Can you work these out from the model? Positions are in its coordinate system, mm. A direction names the side the tool comes from. Coordinates: 2 decimals unless noted, no trailing zeros. Loops run counter-clockwise (first coordinate to the right, second up) from the corner with the lowest first, then second, coordinate; pieces in that order, holes last.
```python
from build123d import *

# Parameters (mm, degrees)
BOSS_EXTRUDE1_DEPTH = 60
SKETCH2_R           = 1.65
SKETCH2_R_2         = 11.5
CUT_EXTRUDE1_DEPTH  = 60
SKETCH3_R           = 1.65
SKETCH3_R_2         = 11.5
CUT_EXTRUDE2_DEPTH  = 60
CUT_EXTRUDE3_START  = -21
SKETCH4_R           = 4
CUT_EXTRUDE3_DEPTH  = 21
SKETCH5_R           = 2.5
CUT_EXTRUDE4_DEPTH  = 6
CUT_EXTRUDE5_DEPTH  = 10
SKETCH9_R           = 5.25
CUT_EXTRUDE7_DEPTH  = 3
CHAMFER1_SIZE       = 1
SKETCH10_W          = 5
SKETCH10_H          = 82
BOSS_EXTRUDE2_DEPTH = 6
FILLET1_R           = 5
SKETCH11_R          = 1.65
CUT_EXTRUDE8_DEPTH  = 10
CUT_EXTRUDE9_DEPTH  = 5
SKETCH13_W          = 82
SKETCH13_H          = 5
BOSS_EXTRUDE3_DEPTH = 6
FILLET2_R           = 5
SKETCH14_R          = 1.5
CUT_EXTRUDE10_DEPTH = 5
CUT_EXTRUDE11_DEPTH = 5


with BuildPart() as part:
    # Sketch1 → Boss-Extrude1 (new body)
    with BuildSketch(Plane(origin=(0, 0, 0), x_dir=(1, 0, 0), z_dir=(0, 1, 0))):
        Polygon((0, 0), (0, -42), (-5, -42), (-5, 40), (0, 40), (0, 5), (82, 5), (82, 0), align=None)
    extrude(amount=BOSS_EXTRUDE1_DEPTH)

    # Sketch2 → Cut-Extrude1 (cut)
    with BuildSketch(Plane.XY):
        with Locations((45.5, 36.5)):
            Circle(SKETCH2_R)
        with Locations((76.5, 36.5)):
            Circle(SKETCH2_R)
        with Locations((76.5, 5.5)):
            Circle(SKETCH2_R)
        with Locations((45.5, 5.5)):
            Circle(SKETCH2_R)
        with Locations((61, 21)):
            Circle(SKETCH2_R_2)
    extrude(amount=-CUT_EXTRUDE1_DEPTH, mode=Mode.SUBTRACT)

    # Sketch3 → Cut-Extrude2 (cut)
    with BuildSketch(Plane(origin=(0, 0, 0), x_dir=(0, 0, -1), z_dir=(1, 0, 0))):
        with Locations((-36.5, 53.5)):
            Circle(SKETCH3_R)
        with Locations((-5.5, 53.5)):
            Circle(SKETCH3_R)
        with Locations((-5.5, 22.5)):
            Circle(SKETCH3_R)
        with Locations((-36.5, 22.5)):
            Circle(SKETCH3_R)
        with Locations((-21, 38)):
            Circle(SKETCH3_R_2)
    extrude(amount=-CUT_EXTRUDE2_DEPTH, mode=Mode.SUBTRACT)

    # Sketch4 → Cut-Extrude3 (cut)
    with BuildSketch(Plane(origin=(0, 0, -5), x_dir=(-1, 0, 0), z_dir=(0, 0, -1)).offset(CUT_EXTRUDE3_START)):
        with Locations((-61, 53)):
            Circle(SKETCH4_R)
        with BuildLine():
            Line((-47.15, 36.5), (-47.15, 41.5))
            ThreePointArc((-47.15, 41.5), (-45.5, 43.15), (-43.85, 41.5))
            Line((-43.85, 41.5), (-43.85, 36.5))
            ThreePointArc((-43.85, 36.5), (-45.5, 34.85), (-47.15, 36.5))
        make_face()
        with BuildLine():
            Line((-78.15, 36.5), (-78.15, 41.5))
            ThreePointArc((-78.15, 41.5), (-76.5, 43.15), (-74.85, 41.5))
            Line((-74.85, 41.5), (-74.85, 36.5))
            ThreePointArc((-74.85, 36.5), (-76.5, 34.85), (-78.15, 36.5))
        make_face()
        with BuildLine():
            Line((-78.15, 5.5), (-78.15, 10.5))
            ThreePointArc((-78.15, 10.5), (-76.5, 12.15), (-74.85, 10.5))
            Line((-74.85, 10.5), (-74.85, 5.5))
            ThreePointArc((-74.85, 5.5), (-76.5, 3.85), (-78.15, 5.5))
        make_face()
        with BuildLine():
            Line((-47.15, 5.5), (-47.15, 10.5))
            ThreePointArc((-47.15, 10.5), (-45.5, 12.15), (-43.85, 10.5))
            Line((-43.85, 10.5), (-43.85, 5.5))
            ThreePointArc((-43.85, 5.5), (-45.5, 3.85), (-47.15, 5.5))
        make_face()
        with BuildLine():
            Line((-72.5, 21), (-72.5, 26))
            ThreePointArc((-72.5, 26), (-61, 37.5), (-49.5, 26))
            Line((-49.5, 26), (-49.5, 21))
            ThreePointArc((-49.5, 21), (-61, 9.5), (-72.5, 21))
        make_face()
    extrude(amount=CUT_EXTRUDE3_DEPTH, mode=Mode.SUBTRACT)

    # Sketch5 → Cut-Extrude4 (cut)
    with BuildSketch(Plane(origin=(0, 0, 0), x_dir=(0, 0, -1), z_dir=(1, 0, 0))):
        with Locations((19, 38)):
            Circle(SKETCH5_R)
    extrude(amount=-CUT_EXTRUDE4_DEPTH, mode=Mode.SUBTRACT)

    # Sketch7 → Cut-Extrude5 (cut)
    with BuildSketch(Plane.ZY.offset(5)):
        with BuildLine():
            Line((-7, 53.85), (-15, 53.85))
            ThreePointArc((-15, 53.85), (-16.65, 55.5), (-15, 57.15))
            Line((-15, 57.15), (-7, 57.15))
            ThreePointArc((-7, 57.15), (-5.35, 55.5), (-7, 53.85))
        make_face()
        with BuildLine():
            Line((-7, 18.85), (-15, 18.85))
            ThreePointArc((-15, 18.85), (-16.65, 20.5), (-15, 22.15))
            Line((-15, 22.15), (-7, 22.15))
            ThreePointArc((-7, 22.15), (-5.35, 20.5), (-7, 18.85))
        make_face()
        with BuildLine():
            Line((-30.930481749, 57.15), (-24.930481749, 57.15))
            ThreePointArc((-24.930481749, 57.15), (-23.280481749, 55.5), (-24.930481749, 53.85))
            Line((-24.930481749, 53.85), (-30.930481749, 53.85))
            ThreePointArc((-30.930481749, 53.85), (-32.580481749, 55.5), (-30.930481749, 57.15))
        make_face()
        with BuildLine():
            Line((-30.930481749, 22.15), (-24.930481749, 22.15))
            ThreePointArc((-24.930481749, 22.15), (-23.280481749, 20.5), (-24.930481749, 18.85))
            Line((-24.930481749, 18.85), (-30.930481749, 18.85))
            ThreePointArc((-30.930481749, 18.85), (-32.580481749, 20.5), (-30.930481749, 22.15))
        make_face()
    extrude(amount=-CUT_EXTRUDE5_DEPTH, mode=Mode.SUBTRACT)

    # Sketch9 → Cut-Extrude7 (cut)
    with BuildSketch(Plane(origin=(0, 0, 0), x_dir=(0, 0, -1), z_dir=(1, 0, 0))):
        with Locations((19, 38)):
            Circle(SKETCH9_R)
    extrude(amount=-CUT_EXTRUDE7_DEPTH, mode=Mode.SUBTRACT)

    # Chamfer1
    chamfer1_edges = [part.edges().sort_by_distance(p)[0] for p in [
        (-3, 38, -16.5),
    ]]
    chamfer(chamfer1_edges, length=CHAMFER1_SIZE)

    # Sketch10 → Boss-Extrude2 (add)
    with BuildSketch(Plane(origin=(0, 60, 0), x_dir=(1, 0, 0), z_dir=(0, 1, 0))):
        with Locations((-2.5, -1)):
            Rectangle(SKETCH10_W, SKETCH10_H)
    extrude(amount=BOSS_EXTRUDE2_DEPTH)

    # Fillet1
    fillet1_edges = [part.edges().sort_by_distance(p)[0] for p in [
        (82, 0, -2.5),
        (-2.5, 66, 42),
        (-2.5, 66, -40),
        (-2.5, 0, 42),
        (-2.5, 0, -40),
    ]]
    fillet(fillet1_edges, radius=FILLET1_R)

    # Sketch11 → Cut-Extrude8 (cut)
    with BuildSketch(Plane.ZY.offset(5)):
        with Locations((21, 62)):
            Circle(SKETCH11_R)
        with Locations((21, 14)):
            Circle(SKETCH11_R)
    extrude(amount=-CUT_EXTRUDE8_DEPTH, mode=Mode.SUBTRACT)

    # Sketch12 → Cut-Extrude9 (cut)
    with BuildSketch(Plane.ZY.offset(5)):
        with BuildLine():
            Line((-15, 41.5), (-7, 41.5))
            ThreePointArc((-7, 41.5), (-3.5, 38), (-7, 34.5))
            Line((-7, 34.5), (-15, 34.5))
            ThreePointArc((-15, 34.5), (-18.5, 38), (-15, 41.5))
        make_face()
    extrude(amount=-CUT_EXTRUDE9_DEPTH, mode=Mode.SUBTRACT)

    # Sketch13 → Boss-Extrude3 (add)
    with BuildSketch(Plane(origin=(0, 60, 0), x_dir=(1, 0, 0), z_dir=(0, 1, 0))):
        with Locations((41, 2.5)):
            Rectangle(SKETCH13_W, SKETCH13_H)
    extrude(amount=BOSS_EXTRUDE3_DEPTH)

    # Fillet2
    fillet2_edges = [part.edges().sort_by_distance(p)[0] for p in [
        (82, 66, -2.5),
    ]]
    fillet(fillet2_edges, radius=FILLET2_R)

    # Sketch14 → Cut-Extrude10 (cut)
    with BuildSketch(Plane.ZY.offset(5)):
        with Locations((-2.5, 62)):
            Circle(SKETCH14_R)
        with Locations((-2.5, 4)):
            Circle(SKETCH14_R)
    extrude(amount=-CUT_EXTRUDE10_DEPTH, mode=Mode.SUBTRACT)

    # Sketch15 → Cut-Extrude11 (cut)
    with BuildSketch(Plane.XY):
        Polygon((0, 63.5), (2, 63.5), (2, 64.75), (4.5, 64.75), (4.5, 63.5), (10, 63.5), (10, 60.5), (4.5, 60.5), (4.5, 59.25), (2, 59.25), (2, 60.5), (0, 60.5), align=None)
        Polygon((4.5, 2.5), (10, 2.5), (10, 5.5), (4.5, 5.5), (4.5, 6.75), (2, 6.75), (2, 5.5), (0, 5.5), (0, 2.5), (2, 2.5), (2, 1.25), (4.5, 1.25), align=None)
    extrude(amount=-CUT_EXTRUDE11_DEPTH, mode=Mode.SUBTRACT)


solid = part.part
```
(1) I'm going to push flat-ended pins straight in: pin 1 (2 mm diameter, centred on x = 15, y = 49.5, fed in from -Z); pin 2 (22.5 mm diameter, centred on y = 38, z = 30, fed in from +X); pin 3 (3 mm diameter, centred on x = 14, y = 44.5, fed in from +Z). Where does each tip first touch, or does it pass through?
Check values:
pin 1: stops at z = -5
pin 2: stops at x = 0
pin 3: stops at z = 0
(2) If we mould it in two halves opening along X, with no side actions, what happens to faces 1 (the flat face through (7, 5.5, -2)), 2 (the cylindrical face through (-2, 64, -39))? For each: released by +X, released by -X, zero draft, split by the parting line, or undercut.
Check values:
face 1: undercut
face 2: zero draft
(3) If I drill on probe 1 along Y at (x, z) = (9, -1); probe 2 along Y at (x, z) = (-2.8, 36.5); probe 3 along X at (y, z) = (41.5, -3), over which ranges is the centre line in solid material (lowest first)?
Check values:
probe 1: y = 0 to 2.5, 5.5 to 60.5, 63.5 to 66
probe 2: y = 0 to 20.85, 24.15 to 51.85, 55.15 to 66
probe 3: x = -5 to 43.85, 47.15 to 74.85, 78.15 to 82
(4) Which directions (+Z, -Z, +X, -X, +Y, -Y) give clear straight access to the entire face, cutting with the end or side of a thin tool? Please do faces 3 (the flat face through (18, 66, -2)), 4 (the flat face through (40, 33, -5)), 5 (the flat face through (-3, 53.85, -11)), 6 (the flat face through (3, 6.75, -2)).
Check values:
face 3: +Z, -Z, +X, -X, +Y
face 4: -Z, +X, +Y, -Y
face 5: +X, -X
face 6: +Z, -Z
(5) I want a section at A-A on z = 21. Write out the boundary of the cut face in (x, y), then the cut area to 3 significant figures.
Check values:
outline: (-5, 0) - (0, 0) - (0, 12.35) - (-5, 12.35) - close; (-5, 15.65) - (0, 15.65) - (0, 26.5) - (-5, 26.5) - close; (-5, 49.5) - (0, 49.5) - (0, 60.35) - (-5, 60.35) - close; (-5, 63.65) - (0, 63.65) - (0, 66) - (-5, 66) - close
area: 182 mm2
(6) I want a section at D-D on x = 26.5. Write out the boundary of the cut face in (y, z).
Check values:
outline: (0, -5) - (66, -5) - (66, 0) - (0, 0) - close
(7) I want a section at C-C on y = 14. Write out the boundary of the cut face in (x, z).
Check values:
outline: (-5, -40) - (0, -40) - (0, -5) - (51.88, -5) - (51.88, 0) - (0, 0) - (0, 19.35) - (-5, 19.35) - close; (-5, 22.65) - (0, 22.65) - (0, 42) - (-5, 42) - close; (70.12, -5) - (82, -5) - (82, 0) - (70.12, 0) - close
(8) I want a section at B-B on z = 5.5. Write out the boundary of the cut face in (x, y), then the cut area to 3 significant figures.
Check values:
outline: (-5, 0) - (0, 0) - (0, 20.85) - (-5, 20.85) - close; (-5, 24.15) - (0, 24.15) - (0, 51.85) - (-5, 51.85) - close; (-5, 55.15) - (0, 55.15) - (0, 66) - (-5, 66) - close
area: 297 mm2
